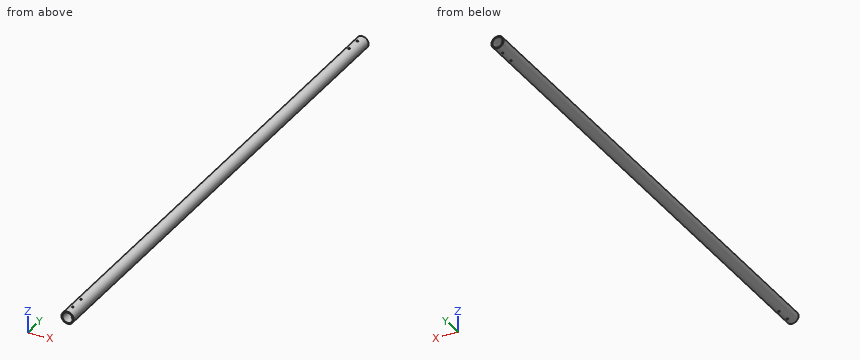
Autodesk Inventor part; units mm, degrees
ref_plane "YZ Plane" through (0, 0, 0) normal (1, 0, 0) x (0, 1, 0)
ref_plane "XZ Plane" through (0, 0, 0) normal (0, 1, 0) x (-1, 0, 0)
ref_plane "XY Plane" through (0, 0, 0) normal (0, 0, 1) x (1, 0, 0)
sketch "Sketch1" plane through (0, 0, 0) normal (0, 1, 0) x (-1, 0, 0)
  circle A0 centre (0, 0) radius 21.082
  circle A1 centre (0, 0) radius 17.526
  dimension "d0" = 42.164
  dimension "d1" = 35.052
extrude "Extrusion1" add sketch "Sketch1" along normal mid plane 1828.8
sketch "Sketch3" plane through (0, 0, 0) normal (0, 0, 1) x (1, 0, 0)
  circle A0 centre (0, 882.65) radius 3.175
  circle A1 centre (0, 831.85) radius 3.175
  line L0 (21.082, 914.4) -> (-21.082, 914.4)
  point P0 (0, 0)
  dimension "d10" = 31.75
  dimension "d11" = 82.55
  dimension "d12" = 6.35
extrude "Extrusion3" cut sketch "Sketch3" against normal through all both and the other way through all
mirror "Mirror1" about plane through (0, 0, 0) normal (0, 1, 0) of "Extrusion3"
properties part number "FE-110-003 Top Bar" material "Aluminum 6061"
Design review of the part built by this model. Coordinates are the model's own, in mm. Give positions to 0.01 mm unless a question says otherwise; leave off trailing zeros. Loops run counter-clockwise (first coordinate to the right, second up) from the corner with the lowest first, then second, coordinate; pieces in that order, holes last. Notation, with made-up numbers: M 38,55 L 89,55 A20 ccw 89,89 Z; hole C -13.5,82.25 d4. An arc over 180 degrees is marked long. Write item = value, one per line.
Q1. Insertion check: pin 1 (3 mm diameter, centred on x = -6.5, y = 708, fed in from -Z); pin 2 (8 mm diameter, centred on x = -7, y = 611.5, fed in from +Z); pin 3 (8 mm diameter, centred on y = -109.5, z = -6.5, fed in from +X). Each pin has a flat end and moves straight along its axis. Give the tip position at first contact, or say it passes through.
Output values:
pin_1 = -20.48
pin_2 = 20.87
pin_3 = 20.93
Q2. To check wall thickness, follow line 1 (Y direction, x = 0, z = 19) (3 decimals); line 2 (X direction, y = -112.5, z = 1.5); line 3 (Z direction, x = 1, y = 801). State the ranges of each line that lie inside material, in increasing order. Write a range as [from, to].
Output values:
line_1 = [-914.4, -885.825], [-879.475, -835.025], [-828.675, 828.675], [835.025, 879.475], [885.825, 914.4]
line_2 = [-21.03, -17.46], [17.46, 21.03]
line_3 = [-21.06, -17.5], [17.5, 21.06]
Q3. We need section B-B (y = 240). Give the boundary of the cut face in (x, z), plus the area to 3 significant figures.
Output values:
outline = C 0,0 d42.16; hole C 0,0 d35.05
area = 431 mm^2
Q4. We need section A-A (z = 0). Give the boundary of the cut face in (x, y), plus the area to 3 significant figures.
Output values:
outline = M -21.08,-914.4 L -17.53,-914.4 L -17.53,914.4 L -21.08,914.4 Z; M 17.53,-914.4 L 21.08,-914.4 L 21.08,914.4 L 17.53,914.4 Z
area = 13,000 mm^2
